Can you work these out from the model? Positions are in its coordinate system, mm. Give positions to 0.01 mm unless a question says otherwise; leave off trailing zeros. Write each loop counter-clockwise with the first axis right and the second up, starting at its lowest first coordinate (ties: lowest second). Pieces come first, ordered by that corner, then holes.
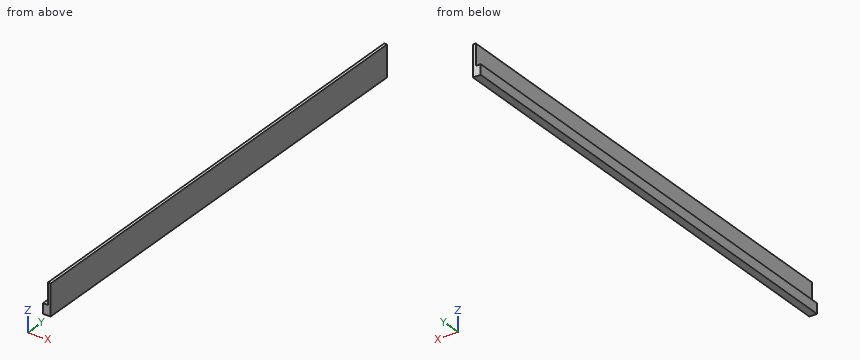
Autodesk Inventor part; units mm, degrees
ref_plane "YZ Plane" through (0, 0, 0) normal (1, 0, 0) x (0, 1, 0)
ref_plane "XZ Plane" through (0, 0, 0) normal (0, 1, 0) x (-1, 0, 0)
ref_plane "XY Plane" through (0, 0, 0) normal (0, 0, 1) x (1, 0, 0)
sketch "Sketch1" plane through (0, 0, 0) normal (0, 1, 0) x (-1, 0, 0)
  point P0 (0, 0)
sketch "Sketch2" plane through (0, 0, 0) normal (0, 1, 0) x (-1, 0, 0)
  line L0 (-0.2857, 31.4286) -> (-6.2857, 31.4286)
  line L1 (-6.2857, 31.4286) -> (-6.2857, -33.5714)
  line L2 (-6.2857, -33.5714) -> (-0.2857, -33.5714)
  line L3 (-0.2857, -33.5714) -> (-0.2857, 31.4286)
  line L4 (9.7143, -12.5714) -> (-0.2857, -12.5714)
  line L5 (-0.2857, -12.5714) -> (-0.2857, -33.5714)
  line L6 (-0.2857, -33.5714) -> (9.7143, -33.5714)
  line L7 (9.7143, -33.5714) -> (9.7143, -12.5714)
  point P0 (0, 0)
  point P1 (-0.2857, -12.5714)
  dimension "d0" = 44
  dimension "d1" = 6
  dimension "d2" = 10
  dimension "d3" = 65
extrude "Extrusion1" add sketch "Sketch2" along normal blind 1000
properties part number "UgolUkrep" material "Aluminum 6061"
1) Suppose I cut it at A-A on y = 349. Write out the boundary of the cut face in (x, z).
Values follow:
outline: (-9.71, -33.57) - (6.29, -33.57) - (6.29, 31.43) - (0.29, 31.43) - (0.29, -12.57) - (-9.71, -12.57) - close
2) Please list where these lines run through material, in increasing order: L1, parallel to Z at x = -6.75, y = 261; L2, parallel to X at y = 947.5, z = 28.5.
Values follow:
L1: z = -33.57 to -12.57
L2: x = 0.29 to 6.29
3) Suppose I cut it at C-C on z = -2.5. Write out the boundary of the cut face in (x, y).
Values follow:
outline: (0.29, 0) - (6.29, 0) - (6.29, 1000) - (0.29, 1000) - close
4) For pin 1 Ø5 at (x, y) = (-3, 605.5) entering from +Z; pin 2 Ø1.5 at (y, z) = (121, 10) entering from -X, each with a flat end and sliding along its axis, tell me the tip position at first contact or that it passes through.
Values follow:
pin 1: stops at z = -12.57
pin 2: stops at x = 0.29
5) Suppose I cut it at B-B on x = -2.5. Write out the boundary of the cut face in (y, z), plus the area to 3 significant figures.
Values follow:
outline: (0, -33.57) - (1000, -33.57) - (1000, -12.57) - (0, -12.57) - close
area: 21,000 mm2
